Could you check a few things on this model? Use its own coordinates, in mm. A direction names the side the tool comes from. Give positions to 0.01 mm unless a question says otherwise; leave off trailing zeros. Loops run counter-clockwise (first coordinate to the right, second up) from the corner with the lowest first, then second, coordinate; pieces in that order, holes last. Notation, with made-up numbers: (22, -38) - (61, -38) arc R26 ccw to (61, -12) - close; hole circle Ø3 at (64.5, -33.5). An arc over 180 degrees is marked (long way). One line per item, written item: value. Start each with the question number.
Q1. For faces 5 (the face through (17, 0, 5)), 6 (the face through (-7, 5, 10)), 7 (the face through (35, 0, 12.6)), 8 (the face through (2, 15, 10)), which set-ups out of +Z, -Z, +X, -X, +Y, -Y let a thin tool reach every point of the face, with its end or its side?
Q2. I want a section at C-C (y = -13). Please give me the cut outline in (x, z), then the cut area to 3 significant figures.
Q3. I want a section at B-B (z = 2). Please give me the cut outline in (x, y), then the cut area to 3 significant figures.
Q4. I'm going to push flat-ended pins straight in: P1, Ø0.8, axis at y = -3.5, z = 18.5, coming from the +X side; P2, Ø4, axis at x = 34.5, y = -9, coming from the +Z side; P3, Ø4, axis at x = 3.5, z = 14.5, coming from the -Y side; P4, Ø3, axis at y = 2, z = 11, coming from the +X side. Where does each tip first touch, or does it pass through?
Q5. If I drill on line 1 (Y direction, x = -7.5, z = 13); line 2 (X direction, y = 4.5, z = 9); line 3 (X direction, y = 13, z = 18), over which ranges is the centre line in solid material (lowest first)? Write a range as from..to.
Q6. I want a section at A-A (y = -3). Please give me the cut outline in (x, z).
Q7. If we mould it in two halves opening along Y, with no side actions, what happens to faces 1 (the face through (40, 25, 15)), 2 (the face through (40, -25, 15)), 3 (the face through (-9, 0, 10)), 4 (the face through (-7, -5, 10))? For each: released by +Y, released by -Y, zero draft, split by the parting line, or undercut.
Q8. I want a section at D-D (x = -19). Please give me the cut outline in (y, z), then the cut area to 3 significant figures.
```python
from build123d import *

# Parameters (mm, degrees)
ESBO_O1_W                = 34
ESBO_O1_H                = 30
ESBO_O1_W_2              = 5
ESBO_O1_H_2              = 10
RESSALTO_EXTRUS_O1_DEPTH = 20.1
ESBO_O2_W                = 10
ESBO_O2_H                = 30
RESSALTO_EXTRUS_O2_DEPTH = 16
RESSALTO_EXTRUS_O3_DEPTH = 50


with BuildPart() as part:
    # Esboço1 → Ressalto-extrusão1 (new body)
    with BuildSketch(Plane.XY):
        Rectangle(ESBO_O1_W, ESBO_O1_H)
        with Locations((-6.5, 0)):
            Rectangle(ESBO_O1_W_2, ESBO_O1_H_2, mode=Mode.SUBTRACT)
    extrude(amount=RESSALTO_EXTRUS_O1_DEPTH)

    # Esboço2 → Ressalto-extrusão2 (add)
    with BuildSketch(Plane(origin=(17, 0, 0), x_dir=(0, 0, -1), z_dir=(1, 0, 0))):
        with Locations((-15.1, 0)):
            Rectangle(ESBO_O2_W, ESBO_O2_H)
    extrude(amount=RESSALTO_EXTRUS_O2_DEPTH)

    # Esboço3 → Ressalto-extrusão3 (add)
    with BuildSketch(Plane(origin=(0, 25, 0), x_dir=(1, 0, 0), z_dir=(0, 1, 0))):
        with BuildLine():
            Line((33, -12.6), (38, -12.6))
            ThreePointArc((38, -12.6), (47.330127019, -15.1), (38, -17.6))
            Line((38, -17.6), (33, -17.6))
            Line((33, -17.6), (33, -12.6))
        make_face()
        with BuildLine():
            Line((-17, -12.6), (-17, -17.6))
            Line((-17, -17.6), (-22, -17.6))
            ThreePointArc((-22, -17.6), (-31.330127019, -15.1), (-22, -12.6))
            Line((-22, -12.6), (-17, -12.6))
        make_face()
    extrude(amount=-RESSALTO_EXTRUS_O3_DEPTH)


solid = part.part
```
Worked answers:
1. face 5: -Z, +X, +Y, -Y
1. face 6: +Z, -Z
1. face 7: -Z, +Y, -Y
1. face 8: +Z, -Z, +Y
2. outline: (-22, 12.6) - (-17, 12.6) - (-17, 0) - (17, 0) - (17, 10.1) - (33, 10.1) - (33, 12.6) - (38, 12.6) arc R5 ccw (long way) to (38, 17.6) - (33, 17.6) - (33, 20.1) - (-17, 20.1) - (-17, 17.6) - (-22, 17.6) arc R5 ccw (long way) to start
2. area: 1,050 mm²
3. outline: (-17, -15) - (17, -15) - (17, 15) - (-17, 15) - close; hole (-9, -5) - (-4, -5) - (-4, 5) - (-9, 5) - close
3. area: 970 mm²
4. P1: stops at x = 46.33
4. P2: stops at z = 20.1
4. P3: stops at y = -15
4. P4: stops at x = 46.6
5. line 1: y = -15..-5, 5..15
5. line 2: x = -17..-9, -4..17
5. line 3: x = -30.4..-22.26, -17..33, 38.26..46.4
6. outline: (-22, 12.6) - (-17, 12.6) - (-17, 0) - (-9, 0) - (-9, 20.1) - (-17, 20.1) - (-17, 17.6) - (-22, 17.6) arc R5 ccw (long way) to start; (-4, 0) - (17, 0) - (17, 10.1) - (33, 10.1) - (33, 12.6) - (38, 12.6) arc R5 ccw (long way) to (38, 17.6) - (33, 17.6) - (33, 20.1) - (-4, 20.1) - close
7. face 1: released by +Y
7. face 2: released by -Y
7. face 3: undercut
7. face 4: undercut
8. outline: (-25, 12.6) - (25, 12.6) - (25, 17.6) - (-25, 17.6) - close
8. area: 250 mm²
